from build123d import *

# Parameters (mm, degrees)
CROQUIS1_R              = 84
CROQUIS1_R_2            = 79
SALIENTE_EXTRUIR1_DEPTH = 2000
CROQUIS2_R              = 84
SALIENTE_EXTRUIR2_DEPTH = 10
SALIENTE_EXTRUIR3_START = -10
CROQUIS3_R              = 84
SALIENTE_EXTRUIR3_DEPTH = 10


with BuildPart() as part:
    # Croquis1 → Saliente-Extruir1 (new body)
    with BuildSketch(Plane(origin=(0, 0, 0), x_dir=(0, 0, -1), z_dir=(1, 0, 0))):
        Circle(CROQUIS1_R)
        Circle(CROQUIS1_R_2, mode=Mode.SUBTRACT)
    extrude(amount=SALIENTE_EXTRUIR1_DEPTH)

    # Croquis2 → Saliente-Extruir2 (add)
    with BuildSketch(Plane.ZY):
        with Locations(Location((0, 0, 0), (0, 0, 180))):
            Circle(CROQUIS2_R)
    extrude(amount=-SALIENTE_EXTRUIR2_DEPTH)

    # Croquis3 → Saliente-Extruir3 (add)
    with BuildSketch(Plane(origin=(2000, 0, 0), x_dir=(0, 0, -1), z_dir=(1, 0, 0)).offset(SALIENTE_EXTRUIR3_START)):
        Circle(CROQUIS3_R)
    extrude(amount=SALIENTE_EXTRUIR3_DEPTH)


solid = part.part
Could you check a few things on this model? Use its own coordinates, in mm. A direction names the side the tool comes from. Give positions to 0.01 mm unless a question says otherwise; leave off trailing zeros. Order: outer loops, then holes, each group sorted by start corner. A loop starts at its lowest first (then second) coordinate and runs counter-clockwise, first axis right, second up.
Item 1: If we mould it in two halves opening along Y, with no side actions, what happens to faces 3 (the face through (986, 25.23, -80.12)), 4 (the face through (10, -1, 1)), 5 (the face through (2000, 1, 1))? For each: pulls with the +Y half, pulls with the -Y half, needs draft (parallel to the pull), parting line crosses it, or undercut.
Item 2: If we section it at C-C, the plane x = 147.5: Write out the boundary of the cut face in (y, z).
Item 3: For faces 1 (the face through (0, 1, 1)), 2 (the face through (986.14, 53.39, 58.23)), which set-ups out of +Z, -Z, +X, -X, +Y, -Y let a thin tool reach every point of the face, with its end or its side?
Item 4: If we section it at A-A, the plane y = 0: Write out the boundary of the cut face in (x, z), plus the area to 3 significant figures.
Item 5: I need wall thicknesses on line 1 (X direction, y = 22.5, z = -30.5); line 2 (Y direction, x = 444, z = 0); line 3 (Y direction, x = 1285.5, z = 33.5). Which ranges of each line are inside material? Lowest first, please.
Item 6: I'm going to push flat-ended pins straight in: pin 1 (5 mm diameter, centred on x = 887.5, z = 4, fed in from +Y); pin 2 (1 mm diameter, centred on x = 1155, y = -6.5, fed in from +Z); pin 3 (6 mm diameter, centred on x = 1629.5, z = 57.5, fed in from +Y). Where does each tip first touch, or does it pass through?
Values:
1. face 3: parting line crosses it
1. face 4: undercut
1. face 5: needs draft
2. outline: circle Ø168 at (0, 0); hole circle Ø158 at (0, 0)
3. face 1: +Z, -Z, -X, +Y, -Y
3. face 2: none
4. outline: (0, -84) - (2000, -84) - (2000, 84) - (0, 84) - close; hole (10, -79) - (1990, -79) - (1990, 79) - (10, 79) - close
4. area: 23,200 mm2
5. line 1: x = 0 to 10, 1990 to 2000
5. line 2: y = -84 to -79, 79 to 84
5. line 3: y = -77.03 to -71.55, 71.55 to 77.03
6. pin 1: stops at y = 83.99
6. pin 2: stops at z = 83.79
6. pin 3: stops at y = 63.92
